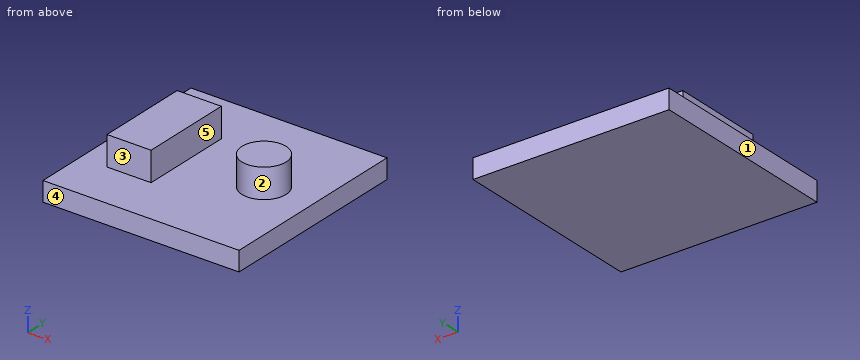
from build123d import *

# Parameters (mm, degrees)
F0_W     = 20
F0_H     = 20
F0_W_2   = 4.5
F0_H_2   = 9.5
F0_R     = 2.25
F1_DEPTH = 2
F2_DEPTH = 5


with BuildPart() as f1:
    # F0 (on Top) → F1 (new body)
    with BuildSketch(Plane.XY):
        Rectangle(F0_W, F0_H)
        with Locations((-5, -0.25)):
            Rectangle(F0_W_2, F0_H_2, mode=Mode.SUBTRACT)
        with Locations((5, 0)):
            Circle(F0_R, mode=Mode.SUBTRACT)
    extrude(amount=F1_DEPTH)

    # F0 (on Top) → F2 (join)
    with BuildSketch(Plane.XY):
        with Locations((-5, -0.25)):
            Rectangle(F0_W_2, F0_H_2)
        with Locations((5, 0)):
            Circle(F0_R)
    extrude(amount=F2_DEPTH)


solid = f1.part
Design review of the part built by this model. Coordinates are the model's own, in mm. Face numbers are marked on the shaded views. A direction names the side the tool comes from. Round coordinates to 2 decimals unless told otherwise and drop trailing zeros. Write each loop counter-clockwise with the first axis right and the second up, starting at its lowest first coordinate (ties: lowest second). Pieces come first, ordered by that corner, then holes. Notation, with made-up numbers: (16.5, -7) - (33.5, -7) arc R13 ccw to (33.5, 9) - close; hole circle Ø5 at (-25.75, 41). An arc over 180 degrees is marked (long way). Use a Markdown table: item, result. Add a question column.
1. We need section C-C (x = 3). State the section outline as (y, z) points, then the cut area to 3 significant figures.
2. We need section A-A (z = 4.4). State the section outline as (x, y) points, then the cut area to 3 significant figures.
3. We need section B-B (y = 0). State the section outline as (x, z) points, then the cut area to 3 significant figures.
4. Clearance check with flat-ended pins moving along their axes: pin 1 (1.5 mm diameter, centred on x = -5, z = 3.5, fed in from -Y); pin 2 (3 mm diameter, centred on x = 4, y = -6.5, fed in from +Z); pin 3 (1.5 mm diameter, centred on y = -2, z = 3.5, fed in from +X). State where each tip first meets the part, or that it passes through.
5. For the marked faces 4 and 5, list the 3-axis set-ups (+Z, -Z, +X, -X, +Y, -Y) from which the entire face can be reached by the end or side of a thin tool; tool diameter is ignored.
6. Wall thickness on probe 1 along X at (y, z) = (-4.5, 3.45); probe 2 along Y at (x, z) = (-4.75, 3.2); probe 3 along Z at (x, y) = (-8.5, -8.25): over which ranges is each line inside the solid? List them lowest first.
7. Mouldability with a two-part tool opening along X and no side actions: class the marked faces 1, 2 and 3 as +X half, -X half, draft (parallel to the pull), parting line (faces both ways), or undercut.
8. We need section D-D (y = -4). State the section outline as (x, z) points, then the cut area to 3 significant figures.
Output:
| question | item | result |
|---|---|---|
| 1 | outline | (-10, 0) - (10, 0) - (10, 2) - (1.03, 2) - (1.03, 5) - (-1.03, 5) - (-1.03, 2) - (-10, 2) - close |
| 1 | area | 46.2 mm2 |
| 2 | outline | (-7.25, -5) - (-2.75, -5) - (-2.75, 4.5) - (-7.25, 4.5) - close; circle Ø4.5 at (5, 0) |
| 2 | area | 58.7 mm2 |
| 3 | outline | (-10, 0) - (10, 0) - (10, 2) - (7.25, 2) - (7.25, 5) - (2.75, 5) - (2.75, 2) - (-2.75, 2) - (-2.75, 5) - (-7.25, 5) - (-7.25, 2) - (-10, 2) - close |
| 3 | area | 67.0 mm2 |
| 4 | pin 1 | stops at y = -5 |
| 4 | pin 2 | stops at z = 2 |
| 4 | pin 3 | stops at x = 6.87 |
| 5 | face 4 | +Z, -Z, +X, -X, -Y |
| 5 | face 5 | +Z, +Y, -Y |
| 6 | probe 1 | x = -7.25 to -2.75 |
| 6 | probe 2 | y = -5 to 4.5 |
| 6 | probe 3 | z = 0 to 2 |
| 7 | face 1 | -X half |
| 7 | face 2 | undercut |
| 7 | face 3 | draft |
| 8 | outline | (-10, 0) - (10, 0) - (10, 2) - (-2.75, 2) - (-2.75, 5) - (-7.25, 5) - (-7.25, 2) - (-10, 2) - close |
| 8 | area | 53.5 mm2 |
